Geometry: see drawing. Coordinates: mm, zero at the bounding-box minimum. A direction names the side the tool comes from. Round coordinates to 2 decimals unless told otherwise and drop trailing zeros. Order: outer loops, then holes, each group sorted by start corner. A loop starts at its lowest first (then second) coordinate and runs counter-clockwise, first axis right, second up. Notation, with made-up numbers: (75, 53.25) -> (101, 53.25) arc R22 cw to (101, 75.25) -> close; hole circle Ø11 at (27, 61). An arc over 180 degrees is marked (long way). Use a Markdown table: item, result.
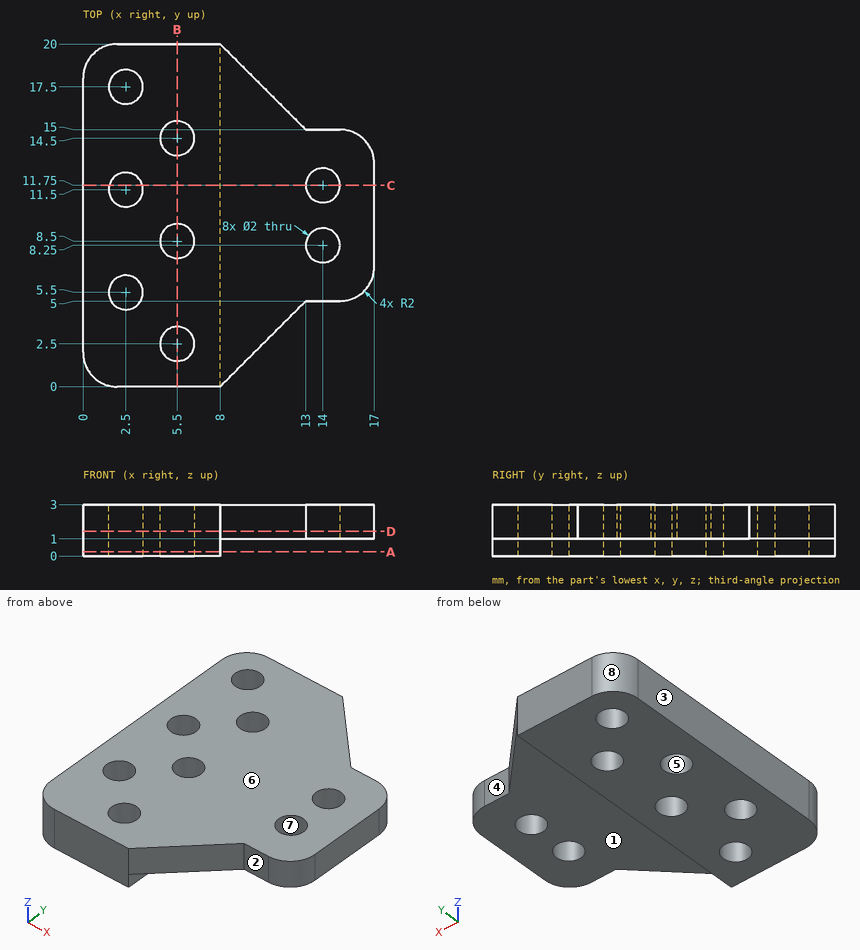
1) Cut plane C-C on y = 11.75. Return loops of the section in (x, z).
Answer key:
| item | result |
|---|---|
| outline | (0, 0) -> (1.53, 0) -> (1.53, 3) -> (0, 3) -> close; (3.47, 0) -> (8, 0) -> (8, 1) -> (13, 1) -> (13, 3) -> (3.47, 3) -> close; (15, 1) -> (17, 1) -> (17, 3) -> (15, 3) -> close |
2) Cut plane D-D on z = 1.45. State how many separate pieces and enclosed holes the cut face has, and give its area (3 significant figures).
Answer key:
| item | result |
|---|---|
| separate pieces | 1 |
| enclosed holes | 8 |
| area | 246 mm^2 |
3) Ray query, probe 1 along Y at (x, z) = (5.5, 2.1); probe 2 along Y at (x, z) = (14, 1.7); probe 3 along Z at (x, y) = (12.5, 7.5). Return the intervals inside material, ascending.
Answer key:
| item | result |
|---|---|
| probe 1 | y = 0 to 1.5, 3.5 to 7.5, 9.5 to 13.5, 15.5 to 20 |
| probe 2 | y = 5 to 7.25, 9.25 to 10.75, 12.75 to 15 |
| probe 3 | z = 1 to 3 |
4) Cut plane A-A on z = 0.25. Return loops of the section in (x, y), and give its area (3 significant figures).
Answer key:
| item | result |
|---|---|
| outline | (0, 2) arc R2 ccw to (2, 0) -> (8, 0) -> (8, 20) -> (2, 20) arc R2 ccw to (0, 18) -> close; hole circle Ø2 at (2.5, 5.5); hole circle Ø2 at (2.5, 11.5); hole circle Ø2 at (2.5, 17.5); hole circle Ø2 at (5.5, 2.5); hole circle Ø2 at (5.5, 8.5); hole circle Ø2 at (5.5, 14.5) |
| area | 139 mm^2 |
5) Cut plane B-B on x = 5.5. Return loops of the section in (y, z), and give its area (3 significant figures).
Answer key:
| item | result |
|---|---|
| outline | (0, 0) -> (1.5, 0) -> (1.5, 3) -> (0, 3) -> close; (3.5, 0) -> (7.5, 0) -> (7.5, 3) -> (3.5, 3) -> close; (9.5, 0) -> (13.5, 0) -> (13.5, 3) -> (9.5, 3) -> close; (15.5, 0) -> (20, 0) -> (20, 3) -> (15.5, 3) -> close |
| area | 42.0 mm^2 |
6) Draft query along X for the marked faces 6, 7 and 8. Return one class per face: released by +X, released by -X, zero draft, split by the parting line, or undercut.
Answer key:
| item | result |
|---|---|
| face 6 | zero draft |
| face 7 | undercut |
| face 8 | released by -X |
7) Set-up query: the marked faces 1, 2, 3, 4 and 5. Return all of +Z, -Z, +X, -X, +Y, -Y with unobstructed straight access to the full face (end or side cutting, diameter ignored); none if empty.
Answer key:
| item | result |
|---|---|
| face 1 | -Z, +X, +Y, -Y |
| face 2 | +Z, -Z, +X, -Y |
| face 3 | +Z, -Z, -X, +Y, -Y |
| face 4 | +Z, -Z, +X, +Y |
| face 5 | +Z, -Z |
8) Contact query for flat-ended pins moving along their axis: P1, Ø1.6, axis at x = 14, z = 2.5, coming from the -Y side; P2, Ø1.2, axis at x = 2.5, y = 17.5, coming from the -Z side; P3, Ø2.5, axis at x = 14, y = 11.75, coming from the -Z side; P4, Ø4, axis at x = 8, y = 6.5, coming from the -Z side. Output: stop coordinate, or through.
Answer key:
| item | result |
|---|---|
| P1 | stops at y = 5 |
| P2 | passes through |
| P3 | stops at z = 1 |
| P4 | stops at z = 0 |
